from build123d import *

# Parameters (mm, degrees)
SKETCH1_W           = 110.344434204
SKETCH1_H           = 110.344434204
SKETCH1_R           = 1.6
SKETCH1_W_2         = 20.7
SKETCH1_H_2         = 41.4
BOSS_EXTRUDE1_DEPTH = 3
SKETCH3_W           = 3.2
SKETCH3_H           = 10.2
SKETCH3_H_2         = 10.372217102
SKETCH3_W_2         = 10.2
SKETCH3_H_3         = 3.2
SKETCH3_H_4         = 30.372217102
CUT_EXTRUDE1_DEPTH  = 4


with BuildPart() as part:
    # Sketch1 → Boss-Extrude1 (new body)
    with BuildSketch(Plane(origin=(0, 0, 0), x_dir=(1, 0, 0), z_dir=(0, 1, 0))):
        with Locations((0, -11.670773756)):
            Rectangle(SKETCH1_W, SKETCH1_H)
        with Locations((-5, 13.9)):
            Circle(SKETCH1_R, mode=Mode.SUBTRACT)
        with Locations((5, 13.9)):
            Circle(SKETCH1_R, mode=Mode.SUBTRACT)
        with Locations((5, -34.6)):
            Circle(SKETCH1_R, mode=Mode.SUBTRACT)
        with Locations((-5, -34.6)):
            Circle(SKETCH1_R, mode=Mode.SUBTRACT)
        with Locations((0, -10.35)):
            Rectangle(SKETCH1_W_2, SKETCH1_H_2, mode=Mode.SUBTRACT)
    extrude(amount=BOSS_EXTRUDE1_DEPTH)

    # Sketch3 → Cut-Extrude1 (cut, through all)
    with BuildSketch(Plane(origin=(0, 0, 0), x_dir=(1, 0, 0), z_dir=(0, 1, 0))):
        with Locations((53.672217102, -1.670773756)):
            Rectangle(SKETCH3_W, SKETCH3_H)
        with Locations((53.672217102, 18.329226244)):
            Rectangle(SKETCH3_W, SKETCH3_H)
        with Locations((53.672217102, 38.415334795)):
            Rectangle(SKETCH3_W, SKETCH3_H_2)
        with Locations((40, -46.292990858)):
            Rectangle(SKETCH3_W_2, SKETCH3_H_3)
        with Locations((53.672217102, -21.670773756)):
            Rectangle(SKETCH3_W, SKETCH3_H)
        with Locations((20, -46.292990858)):
            Rectangle(SKETCH3_W_2, SKETCH3_H_3)
        with Locations((0, -46.292990858)):
            Rectangle(SKETCH3_W_2, SKETCH3_H_3)
        with Locations((-20, -46.292990858)):
            Rectangle(SKETCH3_W_2, SKETCH3_H_3)
        with Locations((-40, -46.292990858)):
            Rectangle(SKETCH3_W_2, SKETCH3_H_3)
        with Locations((-53.672217102, 38.415334795)):
            Rectangle(SKETCH3_W, SKETCH3_H_2)
        with Locations((-53.672217102, 18.329226244)):
            Rectangle(SKETCH3_W, SKETCH3_H)
        with Locations((-53.672217102, -1.670773756)):
            Rectangle(SKETCH3_W, SKETCH3_H)
        with Locations((-53.672217102, -21.670773756)):
            Rectangle(SKETCH3_W, SKETCH3_H)
        with Locations((40, -65.342990858)):
            Rectangle(SKETCH3_W_2, SKETCH3_H_3)
        with Locations((53.672217102, -51.756882307)):
            Rectangle(SKETCH3_W, SKETCH3_H_4)
        with Locations((40, -57.242990858)):
            Rectangle(SKETCH3_W_2, SKETCH3_H_3)
        with Locations((20, -65.342990858)):
            Rectangle(SKETCH3_W_2, SKETCH3_H_3)
        with Locations((0, -65.342990858)):
            Rectangle(SKETCH3_W_2, SKETCH3_H_3)
        with Locations((20, -57.242990858)):
            Rectangle(SKETCH3_W_2, SKETCH3_H_3)
        with Locations((0, -57.242990858)):
            Rectangle(SKETCH3_W_2, SKETCH3_H_3)
        with Locations((-40, -65.342990858)):
            Rectangle(SKETCH3_W_2, SKETCH3_H_3)
        with Locations((-40, -57.242990858)):
            Rectangle(SKETCH3_W_2, SKETCH3_H_3)
        with Locations((-20, -57.242990858)):
            Rectangle(SKETCH3_W_2, SKETCH3_H_3)
        with Locations((-20, -65.342990858)):
            Rectangle(SKETCH3_W_2, SKETCH3_H_3)
        with Locations((-53.672217102, -51.756882307)):
            Rectangle(SKETCH3_W, SKETCH3_H_4)
    extrude(amount=CUT_EXTRUDE1_DEPTH, mode=Mode.SUBTRACT)


solid = part.part
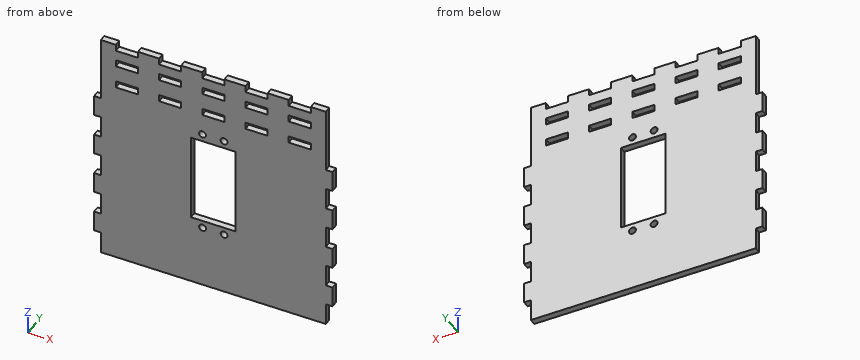
Build history of the part. All positions in model axes, mm. Round coordinates to 2 decimals unless told otherwise and drop trailing zeros. Write each loop counter-clockwise with the first axis right and the second up, starting at its lowest first coordinate (ties: lowest second). Pieces come first, ordered by that corner, then holes. Notation, with made-up numbers: M 74.5,63.25 L 130.5,63.25 A21 cw 130.5,78.25 Z; hole C 56,-7 d2. An arc over 180 degrees is marked long. Answer in a Markdown table with one row per item.
1. Saw through at C-C (z = 11.5). List the corners of the cut face in (x, y), and give its area (3 significant figures).
Geometry check:
| item | result |
|---|---|
| outline | M -55.17,0 L -10.35,0 L -10.35,3 L -55.17,3 Z; M 10.35,0 L 55.17,0 L 55.17,3 L 10.35,3 Z |
| area | 269 mm2 |
2. Flat gauge pins, fed straight in: P1, Ø1.5, axis at y = 1.5, z = -19, coming from the +X side; P2, Ø0.9, axis at y = 2, z = 56.5, coming from the -X side; P3, Ø1.5, axis at x = 41.5, y = 1.5, coming from the +Z side. Where does each tip first touch, or does it go through?
Geometry check:
| item | result |
|---|---|
| P1 | x = 52.07 |
| P2 | x = -52.07 |
| P3 | z = 63.74 |
3. Saw through at B-B (x = 42). List the corners of the cut face in (y, z), and give its area (3 significant figures).
Geometry check:
| item | result |
|---|---|
| outline | M 0,-43.5 L 3,-43.5 L 3,44.69 L 0,44.69 Z; M 0,47.89 L 3,47.89 L 3,55.64 L 0,55.64 Z; M 0,58.84 L 3,58.84 L 3,63.74 L 0,63.74 Z |
| area | 303 mm2 |
4. Saw through at D-D (y = 1.6). State how many separate pieces and enclosed holes the cut face has, and give its area (3 significant figures).
Geometry check:
| item | result |
|---|---|
| separate pieces | 1 |
| enclosed holes | 15 |
| area | 10,400 mm2 |
5. Probe L1, parallel to X at y = 1.8, z = 34.6; L2, parallel to Z at x = 44.5, y = 1.1; L3, parallel to X at y = 2.1, z = -13.9. List the from-to ranges inside material, lowest first. Write a range as [from, to].
Geometry check:
| item | result |
|---|---|
| L1 | [-55.17, -6.6], [-3.4, 3.4], [6.6, 55.17] |
| L2 | [-43.5, 44.69], [47.89, 55.64], [58.84, 63.74] |
| L3 | [-52.07, -6.6], [-3.4, 3.4], [6.6, 52.07] |
6. Saw through at A-A (z = 34.6). List the corners of the cut face in (x, y).
Geometry check:
| item | result |
|---|---|
| outline | M -55.17,0 L -6.6,0 L -6.6,3 L -55.17,3 Z; M -3.4,0 L 3.4,0 L 3.4,3 L -3.4,3 Z; M 6.6,0 L 55.17,0 L 55.17,3 L 6.6,3 Z |
